from build123d import *

# Parameters (mm, degrees)
SKETCH2_W           = 44.45
SKETCH2_H           = 44.45
SKETCH2_R           = 3.175
BOSS_EXTRUDE1_DEPTH = 12.7
FILLET1_R           = 6.35
FILLET2_R           = 1.5875
CHAMFER1_SIZE       = 1.5875


with BuildPart() as part:
    # Sketch2 → Boss-Extrude1 (new body)
    with BuildSketch(Plane(origin=(0, 0, 0), x_dir=(1, 0, 0), z_dir=(0, 1, 0))):
        Rectangle(SKETCH2_W, SKETCH2_H)
        with Locations(Location((-12.7, -12.7, 0), (0, 0, 270))):
            Circle(SKETCH2_R, mode=Mode.SUBTRACT)
        with Locations(Location((12.7, -12.7, 0), (0, 0, 270))):
            Circle(SKETCH2_R, mode=Mode.SUBTRACT)
        with Locations(Location((12.7, 12.7, 0), (0, 0, 270))):
            Circle(SKETCH2_R, mode=Mode.SUBTRACT)
        with Locations(Location((-12.7, 12.7, 0), (0, 0, 270))):
            Circle(SKETCH2_R, mode=Mode.SUBTRACT)
    extrude(amount=BOSS_EXTRUDE1_DEPTH)

    # Fillet1
    fillet1_edges = [part.edges().sort_by_distance(p)[0] for p in [
        (22.225, 6.35, 22.225),
        (-22.225, 6.35, 22.225),
        (-22.225, 6.35, -22.225),
        (22.225, 6.35, -22.225),
    ]]
    fillet(fillet1_edges, radius=FILLET1_R)

    # Fillet2
    fillet2_edges = [part.edges().sort_by_distance(p)[0] for p in [
        (22.225, 12.7, 0),
        (0, 12.7, 22.225),
        (0, 12.7, -22.225),
        (-22.225, 12.7, 0),
        (-20.365128061, 12.7, 20.365128061),
        (20.365128061, 12.7, -20.365128061),
        (-20.365128061, 12.7, -20.365128061),
        (20.365128061, 12.7, 20.365128061),
    ]]
    fillet(fillet2_edges, radius=FILLET2_R)

    # Chamfer1
    chamfer1_edges = [part.edges().sort_by_distance(p)[0] for p in [
        (-12.7, 0, 9.525),
        (-12.7, 12.7, 9.525),
        (12.7, 0, 9.525),
        (12.7, 12.7, 9.525),
        (12.7, 0, -15.875),
        (12.7, 12.7, -15.875),
        (-12.7, 0, -15.875),
        (-12.7, 12.7, -15.875),
        (22.225, 0, 0),
        (0, 0, 22.225),
        (-22.225, 0, 0),
        (0, 0, -22.225),
        (-20.365128061, 0, 20.365128061),
        (20.365128061, 0, -20.365128061),
        (-20.365128061, 0, -20.365128061),
        (20.365128061, 0, 20.365128061),
    ]]
    chamfer(chamfer1_edges, length=CHAMFER1_SIZE)


solid = part.part
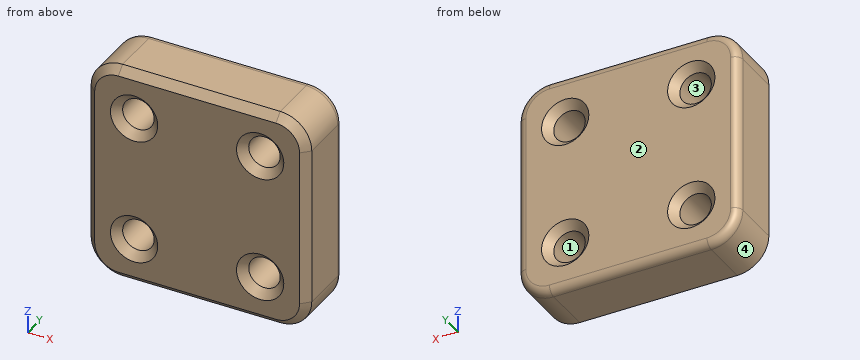
Build history of the part. All positions in model axes, mm. Face numbers are marked on the shaded views. Coordinates: 2 decimals unless noted, no trailing zeros. Write each loop counter-clockwise with the first axis right and the second up, starting at its lowest first coordinate (ties: lowest second). Pieces come first, ordered by that corner, then holes.
(1) Cut at B-B on y = 10. List the corners of the cut face in (x, z) (3 decimals), and give its area (3 significant figures).
(2) Pin check, flat tips, straight feed: pin 1 Ø5.5 at (x, z) = (12.7, 12.7) entering from +Y; pin 2 Ø4 at (x, z) = (-13.5, 10.5) entering from +Y; pin 3 Ø7.5 at (x, z) = (-12.7, 12.7) entering from +Y; pin 4 Ø8.5 at (x, z) = (12.7, -12.7) entering from +Y. Stop position of each tip, or through.
(3) Cut at D-D on y = 1. List the corners of the cut face in (x, z) (1 decimal), and give its area (3 significant figures).
(4) Cut at A-A on z = 12.7. List the corners of the cut face in (x, y) (1 decimal).
(5) Drill centre lines: line 1 (X direction, y = 4.75, z = 12.7) (3 decimals); line 2 (Z direction, x = -15.5, y = 11.25); line 3 (X direction, y = 8, z = -15) (3 decimals). Where is each one in solid material? Low to high.
(6) Mould opens along X. For the marked faces 1, 2, 3 and 4 say: pulls with the +X half, pulls with the -X half, needs draft (parallel to the pull), parting line crosses it, or undercut.
(7) Cut at C-C on x = 12.7. List the corners of the cut face in (y, z) (1 decimal).
Working result:
1. outline: (-22.225, -15.875) arc R6.35 ccw to (-15.875, -22.225) - (15.875, -22.225) arc R6.35 ccw to (22.225, -15.875) - (22.225, 15.875) arc R6.35 ccw to (15.875, 22.225) - (-15.875, 22.225) arc R6.35 ccw to (-22.225, 15.875) - close; hole circle Ø6.35 at (-12.7, -12.7); hole circle Ø6.35 at (-12.7, 12.7); hole circle Ø6.35 at (12.7, -12.7); hole circle Ø6.35 at (12.7, 12.7)
1. area: 1,810 mm2
2. pin 1: passes through
2. pin 2: stops at y = 12.28
2. pin 3: stops at y = 11.69
2. pin 4: stops at y = 12.19
3. outline: (-21.6, -15.9) arc R5.8 ccw to (-15.9, -21.6) - (15.9, -21.6) arc R5.8 ccw to (21.6, -15.9) - (21.6, 15.9) arc R5.8 ccw to (15.9, 21.6) - (-15.9, 21.6) arc R5.8 ccw to (-21.6, 15.9) - close; hole circle Ø7.5 at (-12.7, -12.7); hole circle Ø7.5 at (-12.7, 12.7); hole circle Ø7.5 at (12.7, -12.7); hole circle Ø7.5 at (12.7, 12.7)
3. area: 1,670 mm2
4. outline: (-22.2, 1.6) - (-20.6, 0) - (-17.5, 0) - (-15.9, 1.6) - (-15.9, 11.1) - (-17.5, 12.7) - (-20.6, 12.7) arc R1.6 ccw to (-22.2, 11.1) - close; (-9.5, 1.6) - (-7.9, 0) - (7.9, 0) - (9.5, 1.6) - (9.5, 11.1) - (7.9, 12.7) - (-7.9, 12.7) - (-9.5, 11.1) - close; (15.9, 1.6) - (17.5, 0) - (20.6, 0) - (22.2, 1.6) - (22.2, 11.1) arc R1.6 ccw to (20.6, 12.7) - (17.5, 12.7) - (15.9, 11.1) - close
5. line 1: x = -22.225 to -15.875, -9.525 to 9.525, 15.875 to 22.225
5. line 2: z = -22.22 to -14.47, -10.93 to 10.93, 14.47 to 22.22
5. line 3: x = -22.225 to -14.889, -10.511 to 10.511, 14.889 to 22.225
6. face 1: undercut
6. face 2: needs draft
6. face 3: undercut
6. face 4: pulls with the -X half
7. outline: (0, -20.6) - (1.6, -22.2) - (11.1, -22.2) arc R1.6 ccw to (12.7, -20.6) - (12.7, -17.5) - (11.1, -15.9) - (1.6, -15.9) - (0, -17.5) - close; (0, -7.9) - (1.6, -9.5) - (11.1, -9.5) - (12.7, -7.9) - (12.7, 7.9) - (11.1, 9.5) - (1.6, 9.5) - (0, 7.9) - close; (0, 17.5) - (1.6, 15.9) - (11.1, 15.9) - (12.7, 17.5) - (12.7, 20.6) arc R1.6 ccw to (11.1, 22.2) - (1.6, 22.2) - (0, 20.6) - close
